Geometry check sheet. Reference: drawing and pictorial views, mm from the part's lowest x, y, z. A direction names the side the tool comes from. Coordinates: 2 decimals unless noted, no trailing zeros. Write each loop counter-clockwise with the first axis right and the second up, starting at its lowest first coordinate (ties: lowest second). Pieces come first, ordered by that corner, then holes. Notation, with made-up numbers: (47.25, 13.5) -> (87.25, 13.5) arc R23 cw to (87.25, 48.5) -> close; hole circle Ø9 at (78.25, 74.25). An arc over 180 degrees is marked (long way). Use a Markdown table: item, result.
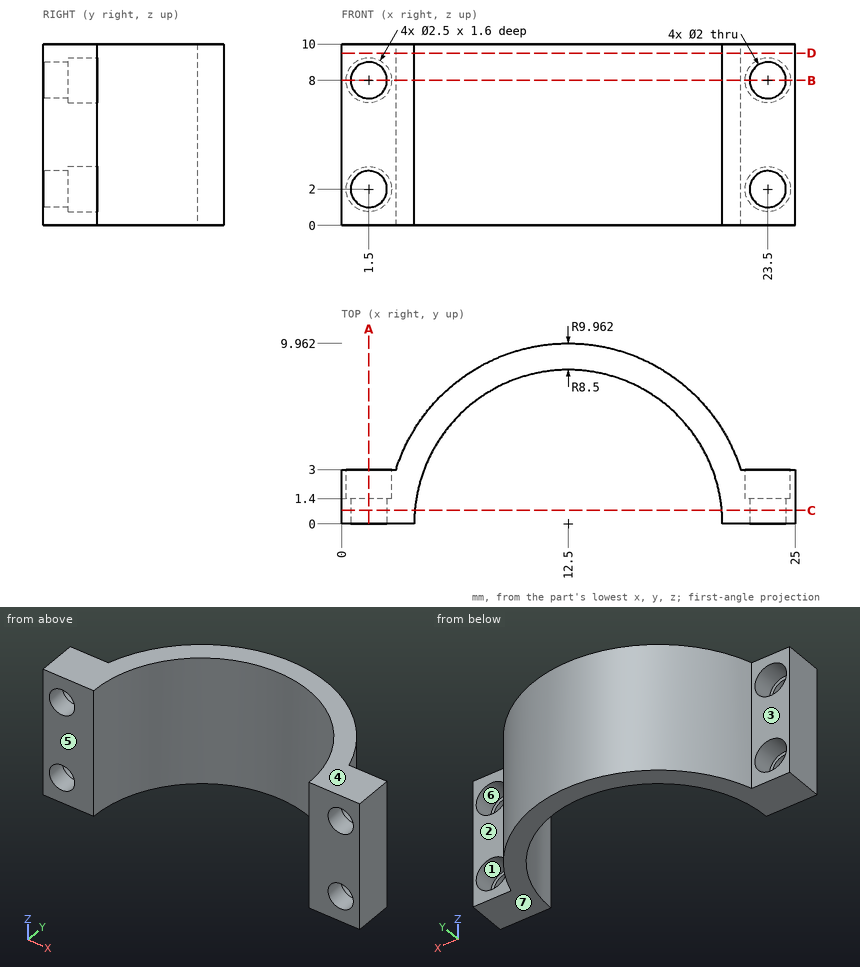
Item 1: Tool access check on the marked faces 1, 2 and 3. Record the directions out of +Z, -Z, +X, -X, +Y, -Y that give a thin tool (end or side, any length) a straight path to the whole face; none if there is none.
Answer block:
| item | result |
|---|---|
| face 1 | +Y |
| face 2 | +Z, -Z, +X, +Y |
| face 3 | +Z, -Z, -X, +Y |
Item 2: Section check D-D on z = 9.5. Record the boundary of the cut face in (x, y) (1 decimal).
Answer block:
| item | result |
|---|---|
| outline | (0, 0) -> (4, 0) arc R8.5 cw to (21, 0) -> (25, 0) -> (25, 3) -> (22, 3) arc R10 ccw to (3, 3) -> (0, 3) -> close |
Item 3: Section check A-A on x = 1.5. Record the boundary of the cut face in (y, z).
Answer block:
| item | result |
|---|---|
| outline | (0, 0) -> (3, 0) -> (3, 0.75) -> (1.4, 0.75) -> (1.4, 1) -> (0, 1) -> close; (0, 3) -> (1.4, 3) -> (1.4, 3.25) -> (3, 3.25) -> (3, 6.75) -> (1.4, 6.75) -> (1.4, 7) -> (0, 7) -> close; (0, 9) -> (1.4, 9) -> (1.4, 9.25) -> (3, 9.25) -> (3, 10) -> (0, 10) -> close |
Item 4: Section check C-C on y = 0.75. Record the boundary of the cut face in (x, z).
Answer block:
| item | result |
|---|---|
| outline | (0, 0) -> (4.03, 0) -> (4.03, 10) -> (0, 10) -> close; (20.97, 0) -> (25, 0) -> (25, 10) -> (20.97, 10) -> close; hole circle Ø2 at (1.5, 2); hole circle Ø2 at (1.5, 8); hole circle Ø2 at (23.5, 2); hole circle Ø2 at (23.5, 8) |
Item 5: Mould release check, pull along Z, two halves, no side actions. Record for the marked faces 4, 5, 6 and 7: +Z half, -Z half, draft (parallel to the pull), parting line (faces both ways), or undercut.
Answer block:
| item | result |
|---|---|
| face 4 | +Z half |
| face 5 | draft |
| face 6 | undercut |
| face 7 | -Z half |
Item 6: Depth check by flat-ended pin: P1, Ø2.5, axis at x = 23.5, z = 5, coming from the +Y side; P2, Ø1, axis at x = 10.5, y = 8.5, coming from the -Z side; P3, Ø0.8, axis at x = 23, z = 7.5, coming from the +Y side; P4, Ø1.5, axis at y = 5, z = 6, coming from the +X side. Enter the tip coordinate at first touch or a pass-through.
Answer block:
| item | result |
|---|---|
| P1 | stops at y = 3 |
| P2 | stops at z = 0 |
| P3 | stops at y = 1.4 |
| P4 | stops at x = 21.51 |
Item 7: Thickness scan on L1, parallel to Z at x = 1.5, y = 1.9; L2, parallel to Z at x = 23.5, y = 1.1; L3, parallel to X at y = 2.6, z = 8. Record the ranges inside material, lowest first. Write a range as [from, to].
Answer block:
| item | result |
|---|---|
| L1 | z = [0, 0.75], [3.25, 6.75], [9.25, 10] |
| L2 | z = [0, 1], [3, 7], [9, 10] |
| L3 | x = [0, 0.25], [2.75, 4.41], [20.59, 22.25], [24.75, 25] |
Item 8: Section check B-B on z = 8. Count the separate pieces of the cut face and the enclosed holes in it.
Answer block:
| item | result |
|---|---|
| separate pieces | 3 |
| enclosed holes | 0 |
